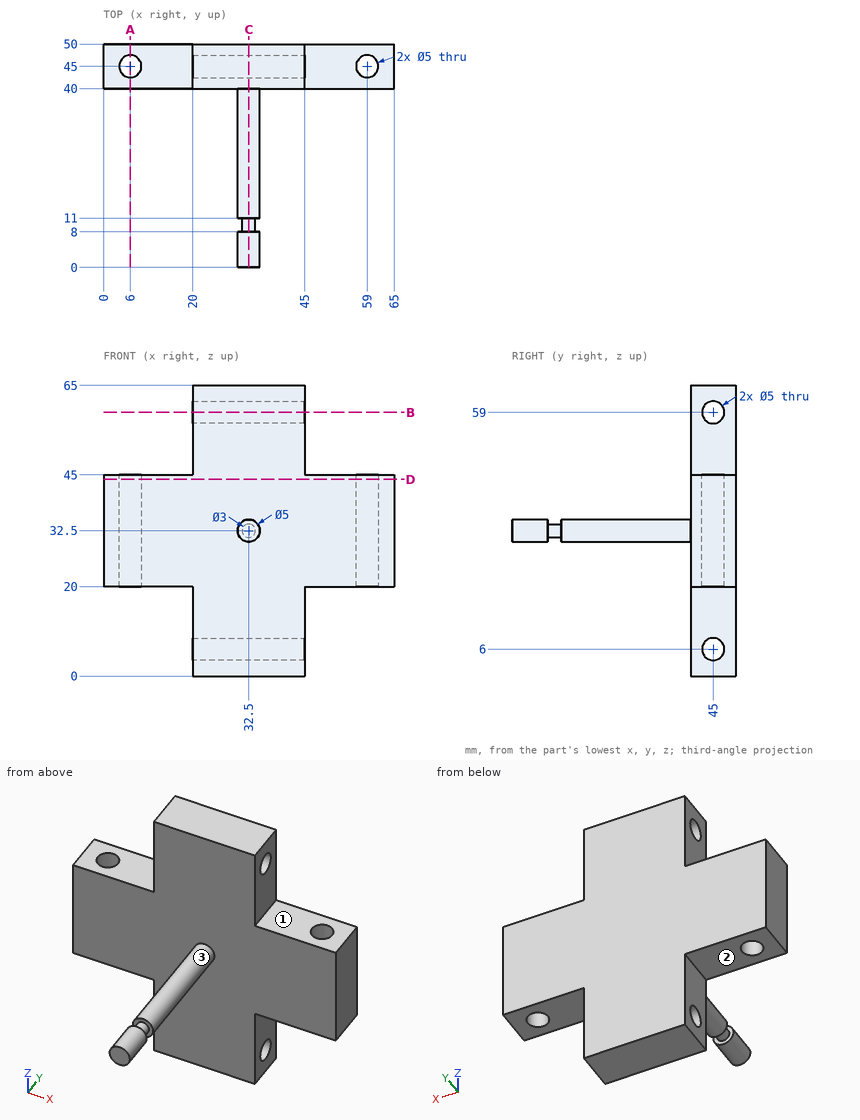
Here's the drawing with two shaded views (mm, measured from the low corner). I have some questions. A direction names the side the tool comes from. Give positions to 0.01 mm unless a question says otherwise; leave off trailing zeros. Write each loop counter-clockwise with the first axis right and the second up, starting at its lowest first coordinate (ties: lowest second). Pieces come first, ordered by that corner, then holes. Notation, with made-up numbers: (49.25, 72) - (67.25, 72) arc R5 cw to (67.25, 80) - close; hole circle Ø10 at (-11, -23). An arc over 180 degrees is marked (long way). Write item = value, one per line. Start each with the question number.
1. On a 3-axis mill with a long thin cutter (end or side, diameter ignored), from which of +Z, -Z, +X, -X, +Y, -Y can I reach the whole of each face in a straight line? I mean the marked faces 1, 2 and 3. Say none if no direction works.
2. Imagine slicing it at C-C (x = 32.5). Please give me the cut outline in (y, z).
3. Imagine slicing it at A-A (x = 6). Please give me the cut outline in (y, z), and give its area (3 significant figures).
4. Imagine slicing it at B-B (z = 59). Please give me the cut outline in (x, y), and give its area (3 significant figures).
5. Imagine slicing it at D-D (z = 44). Please give me the cut outline in (x, y), and give its area (3 significant figures).
6. For pin 1 (6 mm diameter, centred on x = 6, y = 45, fed in from +Z); pin 2 (5 mm diameter, centred on y = 45, z = 15, fed in from +X); pin 3 (1 mm diameter, centred on x = 34.5, z = 19.5, fed in from -Y), each with a flat end and sliding along its axis, tell me the tip position at first contact or that it passes through.
7. Please list where these lines run through material, in increasing order: line 1 (Y direction, x = 6, z = 26); line 2 (Y direction, x = 11.5, z = 31.5); line 3 (X direction, y = 40.5, z = 19).
Worked answers:
q1.face_1 = +Z, +X, +Y, -Y
q1.face_2 = -Z, -X, +Y, -Y
q1.face_3 = -Y
q2.outline = (0, 30) - (8, 30) - (8, 31) - (11, 31) - (11, 30) - (40, 30) - (40, 0) - (50, 0) - (50, 65) - (40, 65) - (40, 35) - (11, 35) - (11, 34) - (8, 34) - (8, 35) - (0, 35) - close; hole circle Ø5 at (45, 6); hole circle Ø5 at (45, 59)
q3.outline = (40, 20) - (42.5, 20) - (42.5, 45) - (40, 45) - close; (47.5, 20) - (50, 20) - (50, 45) - (47.5, 45) - close
q3.area = 125 mm2
q4.outline = (20, 40) - (45, 40) - (45, 42.5) - (20, 42.5) - close; (20, 47.5) - (45, 47.5) - (45, 50) - (20, 50) - close
q4.area = 125 mm2
q5.outline = (0, 40) - (65, 40) - (65, 50) - (0, 50) - close; hole circle Ø5 at (6, 45); hole circle Ø5 at (59, 45)
q5.area = 611 mm2
q6.pin_1 = 45
q6.pin_2 = 45
q6.pin_3 = 40
q7.line_1 = 40 to 42.5, 47.5 to 50
q7.line_2 = 40 to 50
q7.line_3 = 20 to 45
